from build123d import *

# Parameters (mm, degrees)
SKETCH_1_W          = 55.4
SKETCH_1_H          = 13
SKETCH_1_R          = 1.5
SKETCH_1_W_2        = 44
SKETCH_1_H_2        = 4.8
EXTRUDE_1_DEPTH     = 1
SKETCH_2_W          = 55.4
SKETCH_2_H          = 1
EXTRUDE_2_DEPTH     = 7
CUT_EXTRUDE_1_DEPTH = 2
SKETCH_4_R          = 1.5
CUT_EXTRUDE_2_DEPTH = 2
FILLET_1_R          = 0.5
FILLET_2_R          = 1
FILLET_3_R          = 1.5
FILLET_4_R          = 1


with BuildPart() as part:
    # 草图1 → 凸台-拉伸1 (new body)
    with BuildSketch(Plane.XY):
        with Locations((0, 6.5)):
            Rectangle(SKETCH_1_W, SKETCH_1_H)
        with Locations((-24.5, 3)):
            Circle(SKETCH_1_R, mode=Mode.SUBTRACT)
        with Locations((24.5, 3)):
            Circle(SKETCH_1_R, mode=Mode.SUBTRACT)
        with Locations((0, 5.9)):
            Rectangle(SKETCH_1_W_2, SKETCH_1_H_2, mode=Mode.SUBTRACT)
    extrude(amount=EXTRUDE_1_DEPTH)

    # 草图2 → 凸台-拉伸2 (add)
    with BuildSketch(Plane.XY.offset(1)):
        with Locations((0, 12.5)):
            Rectangle(SKETCH_2_W, SKETCH_2_H)
    extrude(amount=EXTRUDE_2_DEPTH)

    # 草图3 → 切除-拉伸1 (cut, through all)
    with BuildSketch(Plane.XZ.offset(-12)):
        Polygon((-27.7, 8), (-27.7, 7), (-10, 8), align=None)
        Polygon((27.7, 8), (27.7, 7), (10, 8), align=None)
    extrude(amount=-CUT_EXTRUDE_1_DEPTH, mode=Mode.SUBTRACT)

    # 草图4 → 切除-拉伸2 (cut, through all)
    with BuildSketch(Plane.XZ.offset(-12)):
        with Locations((-5, 4.25)):
            Circle(SKETCH_4_R)
        with Locations((5, 4.25)):
            Circle(SKETCH_4_R)
    extrude(amount=-CUT_EXTRUDE_2_DEPTH, mode=Mode.SUBTRACT)

    # 圆角1
    fillet_1_edges = [part.edges().sort_by_distance(p)[0] for p in [
        (0, 13, 0),
        (0, 12, 1),
    ]]
    fillet(fillet_1_edges, radius=FILLET_1_R)

    # 圆角2
    fillet_2_edges = [part.edges().sort_by_distance(p)[0] for p in [
        (22, 3.5, 0.5),
        (22, 8.3, 0.5),
        (-22, 8.3, 0.5),
        (-22, 3.5, 0.5),
    ]]
    fillet(fillet_2_edges, radius=FILLET_2_R)

    # 圆角3
    fillet_3_edges = [part.edges().sort_by_distance(p)[0] for p in [
        (27.7, 0, 0.5),
        (-27.7, 0, 0.5),
    ]]
    fillet(fillet_3_edges, radius=FILLET_3_R)

    # 圆角4
    fillet_4_edges = [part.edges().sort_by_distance(p)[0] for p in [
        (-27.7, 12.5, 7),
        (27.7, 12.5, 7),
    ]]
    fillet(fillet_4_edges, radius=FILLET_4_R)


solid = part.part
CAD build for the part. Positions are in the model's coordinates, mm. A direction names the side the tool comes from. Give positions to 0.01 mm unless a question says otherwise; leave off trailing zeros. Write each loop counter-clockwise with the first axis right and the second up, starting at its lowest first coordinate (ties: lowest second). Pieces come first, ordered by that corner, then holes. Notation, with made-up numbers: (57.5, 11.5) - (81.5, 11.5) arc R15 cw to (81.5, 27.5) - close; hole circle Ø9 at (-14.5, 75). An arc over 180 degrees is marked (long way). Put each result on its own line as item: value.
(1) Pull direction X, two halves, no side cores. Call faces 4 (the flat face through (-22, 5.9, 0.5)), 5 (the cylindrical face through (27.434, 12.507, 6.734)), 6 (the flat face through (-0.1, 12.5, 8)), 7 (the cylindrical face through (23, 3.07, 0.49)): released by +X, released by -X, zero draft, split by the parting line, or undercut.
Working result:
face 4: undercut
face 5: released by +X
face 6: zero draft
face 7: undercut
(2) Saw through at C-C (z = 3.75). List the corners of the cut face in (x, y), then the cut area to 3 significant figures.
Working result:
outline: (-27.7, 12) - (-6.41, 12) - (-6.41, 13) - (-27.7, 13) - close; (-3.59, 12) - (3.59, 12) - (3.59, 13) - (-3.59, 13) - close; (6.41, 12) - (27.7, 12) - (27.7, 13) - (6.41, 13) - close
area: 49.7 mm^2
(3) Tool access for faces 1 (the flat face through (-27.7, 8.9, 0.8)), 2 (the flat face through (0, 12, 5)), 3 (the cylindrical face through (21.715, 7.999, 0.507)): list every direction of +Z, -Z, +X, -X, +Y, -Y with a clear straight run to the whole face (end or side of a thin tool).
Working result:
face 1: +Z, -Z, -X, +Y, -Y
face 2: +Z, +X, -X, -Y
face 3: +Z, -Z
(4) Saw through at B-B (x = 8). List the corners of the cut face in (y, z).
Working result:
outline: (0, 0) - (3.5, 0) - (3.5, 1) - (0, 1) - close; (8.3, 0) - (12.5, 0) arc R0.5 ccw to (13, 0.5) - (13, 8) - (12, 8) - (12, 1.5) arc R0.5 cw to (11.5, 1) - (8.3, 1) - close
(5) Saw through at A-A (y = 5). List the corners of the cut face in (x, z).
Working result:
outline: (-27.7, 0) - (-22, 0) - (-22, 1) - (-27.7, 1) - close; (22, 0) - (27.7, 0) - (27.7, 1) - (22, 1) - close
(6) Saw through at D-D (x = 24.5). List the corners of the cut face in (y, z), then the cut area to 3 significant figures.
Working result:
outline: (0, 0) - (1.5, 0) - (1.5, 1) - (0, 1) - close; (4.5, 0) - (12.5, 0) arc R0.5 ccw to (13, 0.5) - (13, 7.18) - (12, 7.18) - (12, 1.5) arc R0.5 cw to (11.5, 1) - (4.5, 1) - close
area: 16.2 mm^2
(7) Drop flat-ended pins along their axis: pin 1 Ø1 at (x, y) = (-6, 6.5) entering from +Z; pin 2 Ø6 at (x, y) = (-13, 5.5) entering from +Z; pin 3 Ø3 at (x, z) = (8.5, 3.5) entering from -Y. Give the stop position or say it passes through.
Working result:
pin 1: through
pin 2: z = 1
pin 3: y = 12
(8) Wall check: L1, parallel to Y at x = -24.5, z = 0.7; L2, parallel to Z at x = 5, y = 12.35; L3, parallel to Y at x = -7, z = 0.5. Give the ranges that are in metal, low to high.
Working result:
L1: 0 to 1.5, 4.5 to 13
L2: 0 to 2.75, 5.75 to 8
L3: 0 to 3.5, 8.3 to 13
